```python
from build123d import *

# Parameters (mm, degrees)
SKETCH_1_W                         = 2
SKETCH_1_H                         = 500
SM_BASE_FLANGE_1_DEPTH             = 210
SM_EDGE_FLANGE_1_STRIP_W           = 11.6
SM_EDGE_FLANGE_1_STRIP_H           = 2
SM_EDGE_FLANGE_1_STRIP_CUT_DEPTH   = 500
SM_EDGE_FLANGE_1_STRIP_2_W         = 11.6
SM_EDGE_FLANGE_1_STRIP_2_H         = 2
SM_EDGE_FLANGE_1_STRIP_CUT_2_DEPTH = 500
SM_EDGE_FLANGE_1_DEPTH             = 500
SM_EDGE_FLANGE_1_BEND_DEPTH        = 500


# Sheet-metal steps are written as plain solids
with BuildPart() as part:
    # Sketch 1 → Базовая кромка1 (new body)
    with BuildSketch(Plane.XY):
        with Locations((1, 250)):
            Rectangle(SKETCH_1_W, SKETCH_1_H)
    extrude(amount=SM_BASE_FLANGE_1_DEPTH)

    # Ребро-кромка1 strip (across the edge) → Ребро-кромка1 strip cut (cut)
    with BuildSketch(Plane(origin=(2, 0, 0), x_dir=(0, 0, 1), z_dir=(0, 1, 0))):
        with Locations((-2, -1)):
            Rectangle(SM_EDGE_FLANGE_1_STRIP_W, SM_EDGE_FLANGE_1_STRIP_H)
    extrude(amount=SM_EDGE_FLANGE_1_STRIP_CUT_DEPTH, mode=Mode.SUBTRACT)

    # Ребро-кромка1 strip 2 (across the edge) → Ребро-кромка1 strip cut 2 (cut)
    with BuildSketch(Plane(origin=(2, 500, 210), x_dir=(0, 0, -1), z_dir=(0, -1, 0))):
        with Locations((-2, -1)):
            Rectangle(SM_EDGE_FLANGE_1_STRIP_2_W, SM_EDGE_FLANGE_1_STRIP_2_H)
    extrude(amount=SM_EDGE_FLANGE_1_STRIP_CUT_2_DEPTH, mode=Mode.SUBTRACT)

    # Ребро-кромка1 section (across the edge) → Ребро-кромка1 (add)
    with BuildSketch(Plane(origin=(2, 0, 0), x_dir=(0, 0, 1), z_dir=(0, 1, 0))):
        with BuildLine():
            Line((0, 1.8), (0, 58))
            Line((0, 58), (2, 58))
            Line((2, 58), (2, 1.8))
            ThreePointArc((2, 1.8), (2.527207794, 0.527207794), (3.8, 0))
            Line((3.8, 0), (3.8, -2))
            ThreePointArc((3.8, -2), (1.112994231, -0.887005769), (0, 1.8))
        make_face()
    extrude(amount=SM_EDGE_FLANGE_1_DEPTH)

    # Ребро-кромка1 section 2 (across the edge) → Ребро-кромка1 bend (add)
    with BuildSketch(Plane(origin=(2, 500, 210), x_dir=(0, 0, -1), z_dir=(0, -1, 0))):
        with BuildLine():
            Line((0, 1.8), (0, 58))
            Line((0, 58), (2, 58))
            Line((2, 58), (2, 1.8))
            ThreePointArc((2, 1.8), (2.527207794, 0.527207794), (3.8, 0))
            Line((3.8, 0), (3.8, -2))
            ThreePointArc((3.8, -2), (1.112994231, -0.887005769), (0, 1.8))
        make_face()
    extrude(amount=SM_EDGE_FLANGE_1_BEND_DEPTH)


solid = part.part
```
Input: part model. Units: mm. Frame: model coordinates. A direction names the side the tool comes from. Give positions to 0.01 mm unless a question says otherwise; leave off trailing zeros. Loops run counter-clockwise (first coordinate to the right, second up) from the corner with the lowest first, then second, coordinate; pieces in that order, holes last. Notation, with made-up numbers: (43, -16.5) -> (80, -16.5) arc R32 cw to (80, 11.5) -> close; hole circle Ø9 at (61.25, 39). An arc over 180 degrees is marked (long way). Use a Markdown table: item, result.
Q1. Ray query, probe 1 along Z at (x, y) = (44, 396.5); probe 2 along X at (y, z) = (362.5, 86). Return the intervals inside material, ascending. Write a range as from..to.
Entries:
| item | result |
|---|---|
| probe 1 | z = 0..2, 208..210 |
| probe 2 | x = 0..2 |
Q2. First-contact query: P1, Ø5, axis at y = 305, z = 157, coming from the +X side. Flat tip, straight axial feed; report the tip coordinate or a pass-through.
Entries:
| item | result |
|---|---|
| P1 | stops at x = 2 |
Q3. Pull-direction query (Z, two-part tool) for faces 3 (the flat face through (32, 246, 2)), 4 (the flat face through (0, 247, 104)), 5 (the flat face through (32, 254, 210)); classes: pulls with the +Z half, pulls with the -Z half, needs draft (parallel to the pull), parting line crosses it, or undercut.
Entries:
| item | result |
|---|---|
| face 3 | undercut |
| face 4 | needs draft |
| face 5 | pulls with the +Z half |
Q4. Section query A-A, the plane x = 36.5. Return the cut outline in (y, z), plus the area to 3 significant figures.
Entries:
| item | result |
|---|---|
| outline | (0, 0) -> (500, 0) -> (500, 2) -> (0, 2) -> close; (0, 208) -> (500, 208) -> (500, 210) -> (0, 210) -> close |
| area | 2,000 mm² |
Q5. Access query for faces 1 (the flat face through (2, 247, 104)), 2 (the flat face through (1, 500, 105)). Directions: +Z, -Z, +X, -X, +Y, -Y. A direction counts if a zero-diameter tool reaches every point of the face in a straight line with its end or side. Return the directions, or none.
Entries:
| item | result |
|---|---|
| face 1 | +X, +Y, -Y |
| face 2 | +Z, -Z, +X, -X, +Y |
Q6. Section query C-C, the plane z = 120.5. Return the cut outline in (x, y).
Entries:
| item | result |
|---|---|
| outline | (0, 0) -> (2, 0) -> (2, 500) -> (0, 500) -> close |
Q7. Section query B-B, the plane y = 38. Return the cut outline in (x, z), plus the area to 3 significant figures.
Entries:
| item | result |
|---|---|
| outline | (0, 3.8) arc R3.8 ccw to (3.8, 0) -> (60, 0) -> (60, 2) -> (3.8, 2) arc R1.8 cw to (2, 3.8) -> (2, 206.2) arc R1.8 cw to (3.8, 208) -> (60, 208) -> (60, 210) -> (3.8, 210) arc R3.8 ccw to (0, 206.2) -> close |
| area | 647 mm² |
